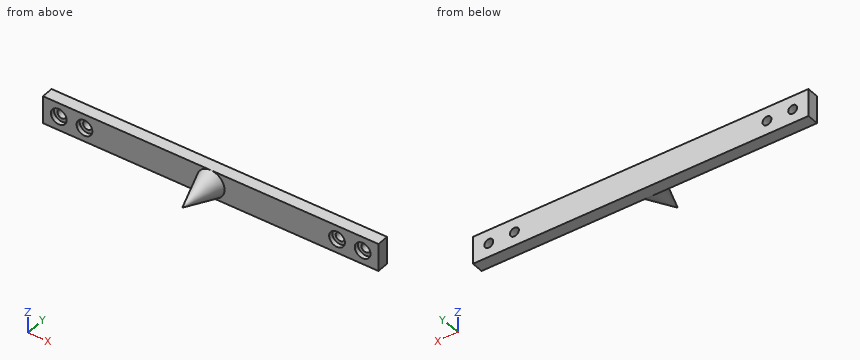
from build123d import *

# Parameters (mm, degrees)
SKIZZE1_W                                           = 170
SKIZZE1_H                                           = 14
AUFSATZ_LINEAR_AUSTRAGEN1_DEPTH                     = 6
STIRNSENKUNG_F_R_M4_SENKSCHRAUBE_KOPF_B_D           = 4.5
STIRNSENKUNG_F_R_M4_SENKSCHRAUBE_KOPF_B_CBORE_D     = 8
STIRNSENKUNG_F_R_M4_SENKSCHRAUBE_KOPF_B_CBORE_DEPTH = 2.2


with BuildPart() as part:
    # Skizze1 → Aufsatz-Linear austragen1 (new body)
    with BuildSketch(Plane(origin=(0, 0, 0), x_dir=(1, 0, 0), z_dir=(0, 1, 0))):
        Rectangle(SKIZZE1_W, SKIZZE1_H)
    extrude(amount=AUFSATZ_LINEAR_AUSTRAGEN1_DEPTH)

    # Stirnsenkung für M4 Senkschraube (Kopf Button)1 (through all)
    with Locations(Plane(origin=(-77, 0, 0), x_dir=(0, 0, -1), z_dir=(0, -1, 0))):
        with Locations((0, 0), (0, 13), (0, 141), (0, 154)):
            CounterBoreHole(STIRNSENKUNG_F_R_M4_SENKSCHRAUBE_KOPF_B_D / 2, STIRNSENKUNG_F_R_M4_SENKSCHRAUBE_KOPF_B_CBORE_D / 2, STIRNSENKUNG_F_R_M4_SENKSCHRAUBE_KOPF_B_CBORE_DEPTH)

    # Skizze3 → Rotation1 (revolve)
    with BuildSketch(Plane.XY):
        Polygon((-7, 0), (0, -20), (0, 0), align=None)
    revolve(axis=Axis((0, 32.961151518, 0), (0, -1, 0)))


solid = part.part
Model file for the job. Use its own axes, mm. Give positions to 0.01 mm unless a question says otherwise; leave off trailing zeros. Order: outer loops, then holes, each group sorted by start corner. A loop starts at its lowest first (then second) coordinate and runs counter-clockwise, first axis right, second up. Notation, with made-up numbers: (40.25, -20.5) - (78.25, -20.5) arc R31 cw to (78.25, 12.5) - close; hole circle Ø8 at (40.5, 87). An arc over 180 degrees is marked (long way). Write item = value, one per line. Start each with the question number.
1. Cut at B-B, the plane x = 50. List the corners of the cut face in (y, z), and give its area (3 significant figures).
2. Drop flat-ended pins along their axis: P1, Ø1, axis at y = -10, z = 1, coming from the -X side; P2, Ø2.5, axis at x = 64.5, z = -2, coming from the -Y side; P3, Ø7, axis at x = -40.5, z = 2.5, coming from the -Y side. Give the stop position or say it passes through.
3. Probe line 1 along X through (y, z) = (0.95, 0); line 2 along X through (y, z) = (3.3, 0); line 3 along Y through (x, z) = (64, -2.75). List the from-to ranges inside material, lowest first.
4. Cut at A-A, the plane x = -64. List the corners of the cut face in (y, z), and give its area (3 significant figures).
5. Cut at C-C, the plane y = -15.75. List the corners of the cut face in (x, z) (1 decimal).
Taken from the geometry:
q1.outline = (0, -7) - (6, -7) - (6, 7) - (0, 7) - close
q1.area = 84.0 mm²
q2.P1 = -3.57
q2.P2 = 2.2
q2.P3 = 0
q3.line_1 = -85 to -81, -73 to -68, -60 to 60, 68 to 73, 81 to 85
q3.line_2 = -85 to -79.25, -74.75 to -66.25, -61.75 to 61.75, 66.25 to 74.75, 79.25 to 85
q3.line_3 = 2.2 to 6
q4.outline = (0, -7) - (6, -7) - (6, -2.25) - (2.2, -2.25) - (2.2, -4) - (0, -4) - close; (0, 4) - (2.2, 4) - (2.2, 2.25) - (6, 2.25) - (6, 7) - (0, 7) - close
q4.area = 49.3 mm²
q5.outline = circle Ø3 at (0, 0)
